```python
from build123d import *

# Parameters (mm, degrees)
F0_W     = 25.4
F0_H     = 25.4
F1_DEPTH = 25.4
F3_DEPTH = 25.4
F4_R     = 0.508


with BuildPart() as f1:
    # F0 (on Front) → F1 (new body)
    with BuildSketch(Plane.XZ):
        with Locations((12.7, 12.7)):
            Rectangle(F0_W, F0_H)
    extrude(amount=F1_DEPTH)

    # F2 (on face) → F3 (cut)
    with BuildSketch(Plane.YZ.offset(25.4)):
        Polygon((0, 25.4), (-25.4, 25.4), (0, 0), align=None)
    extrude(amount=-F3_DEPTH, mode=Mode.SUBTRACT)

    # F4
    f4_edges = [f1.edges().sort_by_distance(p)[0] for p in [
        (0, -25.4, 12.7),
        (12.7, -25.4, 0),
        (25.4, -25.4, 12.7),
        (12.7, -25.4, 25.4),
        (25.4, -12.7, 12.7),
        (25.4, -12.7, 0),
        (12.7, 0, 0),
        (0, -12.7, 12.7),
        (0, -12.7, 0),
    ]]
    fillet(f4_edges, radius=F4_R)


solid = f1.part
```
The listing builds one solid part. Answer for the finished solid, in the listing's coordinates (mm). Give positions to 0.01 mm unless a question says otherwise; leave off trailing zeros. Order: outer loops, then holes, each group sorted by start corner. A loop starts at its lowest first (then second) coordinate and runs counter-clockwise, first axis right, second up. Notation, with made-up numbers: (5.5, -4) - (23.5, -4) arc R25 ccw to (23.5, 21) - close; hole circle Ø1 at (84.25, 33.25). An arc over 180 degrees is marked (long way). Use one line per item in the form item = value. Start each with the question number.
(1) Flat-ended cylindrical pins translate along their axes: pin 1 Ø1.5 at (x, y) = (17.5, -10.5) entering from +Z; pin 2 Ø12 at (y, z) = (-8, 21.5) entering from -X; pin 3 Ø1 at (x, z) = (21.5, 2.5) entering from +Y; pin 4 Ø12 at (x, z) = (11, 17.5) entering from +Y. Find the tip coordinate at first contact, or state that the pin passes through.
(2) A cutting plane is placed at A-A, the plane x = 3.5. Write down the section's boundary in (y, z), then the cut area to 3 significant figures.
(3) Consider line 1 (Y direction, x = 18.25, z = 19.5); line 2 (Z direction, x = 23.5, y = -6.25); line 3 (Y direction, x = 2, z = 16.75). Determine where each line is inside the solid, lowest interval first. Write a range as from..to.
Ans:
q1.pin_1 = 11.25
q1.pin_2 = through
q1.pin_3 = -2
q1.pin_4 = -11.5
q2.outline = (-25.4, 0.51) arc R0.51 ccw to (-24.89, 0) - (-1.23, 0) arc R0.51 ccw to (-0.87, 0.87) - (-24.53, 24.53) arc R0.51 ccw to (-25.4, 24.17) - close
q2.area = 322 mm^2
q3.line_1 = -25.4..-19.5
q3.line_2 = 0..6.25
q3.line_3 = -25.4..-16.75
